Autodesk Inventor part; units mm, degrees
ref_plane "YZ Plane" through (0, 0, 0) normal (1, 0, 0) x (0, 1, 0)
ref_plane "XZ Plane" through (0, 0, 0) normal (0, 1, 0) x (-1, 0, 0)
ref_plane "XY Plane" through (0, 0, 0) normal (0, 0, 1) x (1, 0, 0)
sketch "Sketch1" plane through (0, 0, 0) normal (1, 0, 0) x (0, 1, 0)
  line L0 (0, 0) -> (63.5, 0)
  line L1 (76.2, -12.7) -> (76.2, -38.1)
  line L2 (63.5, -50.8) -> (0, -50.8)
  line L3 (0, -50.8) -> (0, 0)
  circle A0 centre (50.8, -25.4) radius 16.002
  arc A1 (76.2, -12.7) -> (63.5, 0) centre (63.5, -12.7) ccw
  arc A2 (63.5, -50.8) -> (76.2, -38.1) centre (63.5, -38.1) ccw
  point P0 (76.2, -50.8)
  point P1 (76.2, 0)
  dimension "d1" = 76.2
  dimension "d2" = 50.8
  dimension "d6" = 32.004
  dimension "d7" = 12.7
extrude "Extrusion1" add sketch "Sketch1" along normal blind 25.4
ref_plane "Work Plane1" through (0, 0, -50.8) normal (0, -1, 0) x (1, 0, 0)
sketch "Sketch2" plane through (0, 0, -50.8) normal (0, -1, 0) x (1, 0, 0)
  line L0 (0, 50.8) -> (25.4, 50.8)
  line L1 (25.4, 50.8) -> (25.4, 63.5)
  line L2 (25.4, 63.5) -> (0, 63.5)
  line L3 (0, 63.5) -> (0, 50.8)
  line L4 (0, 50.8) -> (0, 0)
  line L5 (0, 0) -> (25.4, 0)
  line L6 (25.4, 0) -> (25.4, -12.7)
  line L7 (25.4, -12.7) -> (0, -12.7)
  line L8 (0, -12.7) -> (0, 0)
  circle A0 centre (12.7, 57.15) radius 3.9687
  circle A1 centre (12.7, -6.35) radius 3.9688
  dimension "d11" = 25.4
  dimension "d12" = 25.4
  dimension "d13" = 12.7
  dimension "d14" = 12.7
  dimension "d15" = 7.9375
  dimension "d16" = 7.9375
extrude "Extrusion2" add sketch "Sketch2" against normal blind 19.05 contours L3 L2 L1 L0 | L5 L6 L7 L8 | A0 | A1
sketch "Sketch3" plane through (0, 19.05, -50.8) normal (0, 1, 0) x (1, 0, 0)
  line L0 (0, -63.5) -> (25.4, -63.5)
  circle A0 centre (12.7, -57.15) radius 3.9688
  line L1 (25.4, 12.7) -> (0, 12.7)
  circle A1 centre (12.7, 6.35) radius 3.9688
  point P0 (0, -50.8)
  dimension "d20" = 7.9375
hole "Hole1" at (12.7, 19.05, -57.15) direction (0, -1, 0) diameter 6.4008 end through all counterbore diameter 7.9375 counterbore depth 6.35
hole "Hole2" at (12.7, 19.05, 6.35) direction (0, -1, 0) diameter 6.4008 end through all counterbore diameter 7.9375 counterbore depth 6.35
equation "\"d23\" = d12"
equation "\"d30\" = d12"
properties part number "motor_mount_wrist"
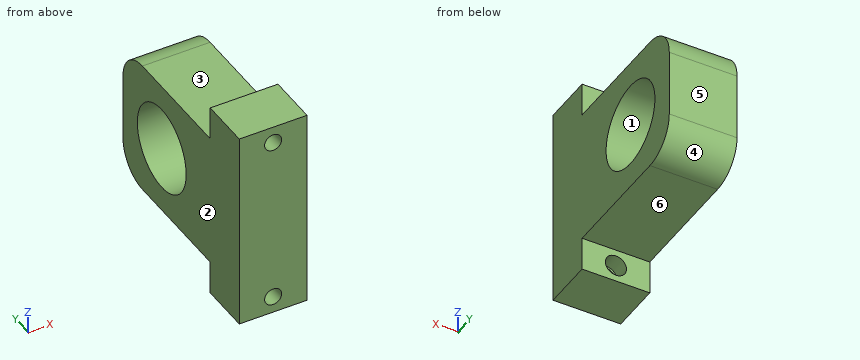
Can you work these out from the model? Positions are in its coordinate system, mm. Face numbers are marked on the shaded views. A direction names the side the tool comes from. Round coordinates to 2 decimals unless told otherwise and drop trailing zeros. Loops run counter-clockwise (first coordinate to the right, second up) from the corner with the lowest first, then second, coordinate; pieces in that order, holes last. Notation, with made-up numbers: (34, 52) -> (82, 52) arc R29 cw to (82, 89) -> close; hole circle Ø7 at (34.5, 81). An arc over 180 degrees is marked (long way). One line per item, written item: value. Start each with the question number.
1. If I drill on probe 1 along X at (y, z) = (3.75, 6.35); probe 2 along X at (y, z) = (13.5, -57); probe 3 along Z at (x, y) = (12.7, 10.25), over which ranges is the centre line in solid material (lowest first)?
2. If we section it at B-B, the plane z = 6.35: Write out the boundary of the cut face in (x, y), then the cut area to 3 significant figures.
3. For pin 1 (6.5 mm diameter, centred on x = 12.7, z = 6.35, fed in from -Y); pin 2 (12.5 mm diameter, centred on x = 9, y = 40, fed in from +Z); pin 3 (10 mm diameter, centred on x = 13.5, z = -58.5, fed in from +Y); pin 4 (8 mm diameter, centred on x = 13, z = -7.5, fed in from +Y), each with a flat end and sliding along its axis, tell me the tip position at first contact or that it passes through.
4. For the marked faces 5 and 6, which set-ups out of +Z, -Z, +X, -X, +Y, -Y let a thin tool reach every point of the face, with its end or its side?
5. If we section it at D-D, the plane y = 11: Write out the boundary of the cut face in (x, z).
6. If we mould it in two halves opening along Z, with no side actions, what happens to the marked faces 1, 2, 3 and 4? For each: pulls with the +Z half, pulls with the -Z half, needs draft (parallel to the pull), parting line crosses it, or undercut.
7. If we section it at A-A, the plane y = 50.8: Write out the boundary of the cut face in (x, z), then the cut area to 3 significant figures.
8. If we section it at C-C, the plane x = 12.7: Write out the boundary of the cut face in (y, z), then the cut area to 3 significant figures.
Calculated:
1. probe 1: x = 0 to 9.5, 15.9 to 25.4
1. probe 2: x = 0 to 8.73, 16.67 to 25.4
1. probe 3: z = -63.5 to -60.35, -53.95 to 3.15, 9.55 to 12.7
2. outline: (0, 0) -> (9.5, 0) -> (9.5, 12.7) -> (8.73, 12.7) -> (8.73, 19.05) -> (0, 19.05) -> close; (15.9, 0) -> (25.4, 0) -> (25.4, 19.05) -> (16.67, 19.05) -> (16.67, 12.7) -> (15.9, 12.7) -> close
2. area: 352 mm²
3. pin 1: stops at y = 0
3. pin 2: stops at z = 0
3. pin 3: stops at y = 19.05
3. pin 4: stops at y = 76.14
4. face 5: +Z, -Z, +X, -X, +Y
4. face 6: -Z, +X, -X, +Y
5. outline: (0, -63.5) -> (25.4, -63.5) -> (25.4, 12.7) -> (0, 12.7) -> close; hole circle Ø6.4 at (12.7, -57.15); hole circle Ø6.4 at (12.7, 6.35)
6. face 1: undercut
6. face 2: needs draft
6. face 3: pulls with the +Z half
6. face 4: pulls with the -Z half
7. outline: (0, -50.8) -> (25.4, -50.8) -> (25.4, -41.4) -> (0, -41.4) -> close; (0, -9.4) -> (25.4, -9.4) -> (25.4, 0) -> (0, 0) -> close
7. area: 477 mm²
8. outline: (0, -63.5) -> (19.05, -63.5) -> (19.05, -61.12) -> (12.7, -61.12) -> (12.7, -60.35) -> (0, -60.35) -> close; (0, -53.95) -> (12.7, -53.95) -> (12.7, -53.18) -> (19.05, -53.18) -> (19.05, -50.8) -> (63.5, -50.8) arc R12.7 ccw to (76.2, -38.1) -> (76.2, -12.7) arc R12.7 ccw to (63.5, 0) -> (19.05, 0) -> (19.05, 2.38) -> (12.7, 2.38) -> (12.7, 3.15) -> (0, 3.15) -> close; (0, 9.55) -> (12.7, 9.55) -> (12.7, 10.32) -> (19.05, 10.32) -> (19.05, 12.7) -> (0, 12.7) -> close; hole circle Ø32 at (50.8, -25.4)
8. area: 3,220 mm²
